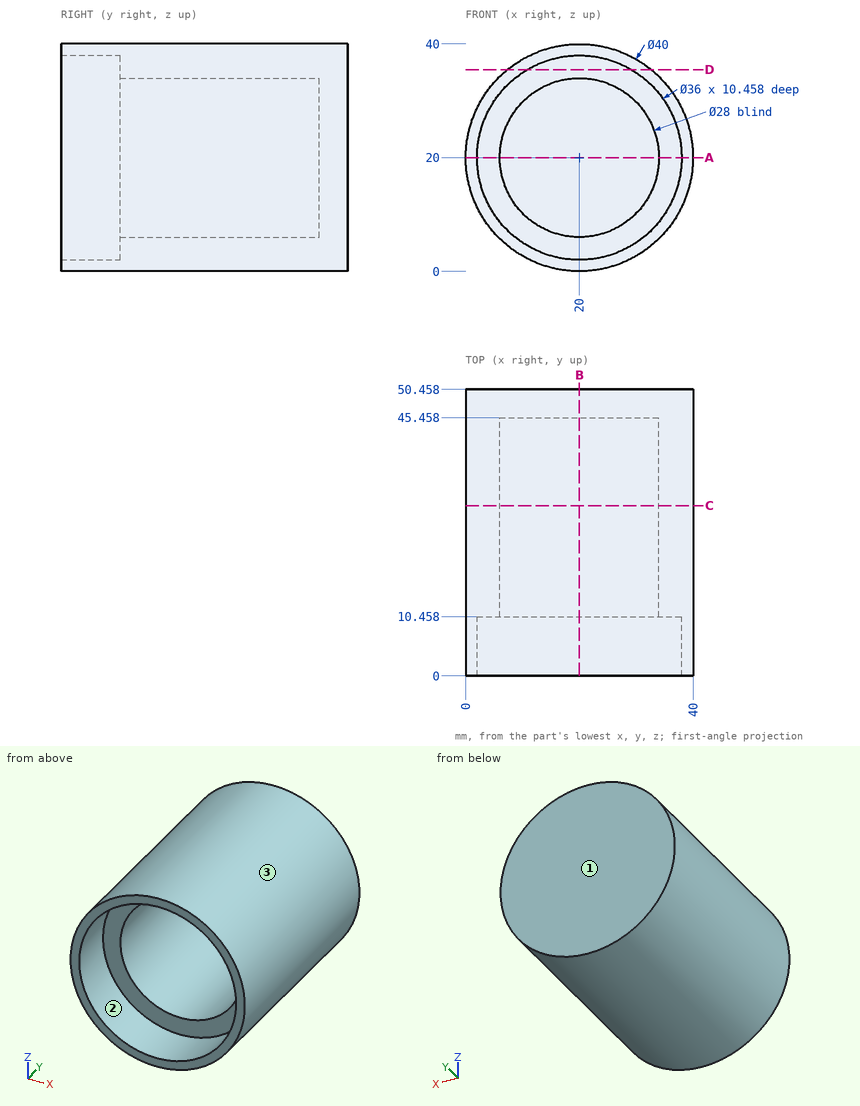
For this review, use the dimensioned drawing (mm, ordinates from the lowest corner) and the shaded views. Give positions to 0.01 mm unless a question says otherwise; leave off trailing zeros. Write each loop counter-clockwise with the first axis right and the second up, starting at its lowest first coordinate (ties: lowest second). Pieces come first, ordered by that corner, then holes. Notation, with made-up numbers: M -2.5,48 L 20.5,48 A15 ccw 20.5,69 Z; hole C -32.75,-38 d10. An arc over 180 degrees is marked long. Write item = value, one per line. Start each with the question number.
Q1. We need section D-D (z = 35.5). State the section outline as (x, y) points, plus the area to 3 significant figures.
Q2. For line 1 (X direction, y = 42, z = 20); line 2 (Y direction, x = 24.5, z = 15); line 3 (X direction, y = 13, z = 25.5), list the stretches that pass through material, from the lowest coordinate up.
Q3. Clearance check with flat-ended pins moving along their axes: pin 1 (6 mm diameter, centred on y = 42.5, z = 24, fed in from +X) (3 decimals); pin 2 (22.5 mm diameter, centred on x = 17, z = 16, fed in from -Y); pin 3 (1 mm diameter, centred on x = 11.5, z = 21, fed in from -Y). State where each tip first meets the part, or that it passes through.
Q4. We need section B-B (x = 20). State the section outline as (y, z) points, plus the area to 3 significant figures.
Q5. Mouldability with a two-part tool opening along X and no side actions: class the marked faces 1, 2 and 3 as released by +X, released by -X, zero draft, split by the parting line, or undercut.
Q6. We need section C-C (y = 30). State the section outline as (x, z) points, plus the area to 3 significant figures.
Q7. We need section A-A (z = 20). State the section outline as (x, y) points, plus the area to 3 significant figures.
Result set:
q1.outline = M 7.36,0 L 10.85,0 L 10.85,10.46 L 29.15,10.46 L 29.15,0 L 32.64,0 L 32.64,50.46 L 7.36,50.46 Z
q1.area = 1,080 mm2
q2.line_1 = 0 to 6, 34 to 40
q2.line_2 = 45.46 to 50.46
q2.line_3 = 0.77 to 7.13, 32.87 to 39.23
q3.pin_1 = 39.975
q3.pin_2 = 10.46
q3.pin_3 = 45.46
q4.outline = M 0,0 L 50.46,0 L 50.46,40 L 0,40 L 0,38 L 10.46,38 L 10.46,34 L 45.46,34 L 45.46,6 L 10.46,6 L 10.46,2 L 0,2 Z
q4.area = 662 mm2
q5.face_1 = zero draft
q5.face_2 = undercut
q5.face_3 = split by the parting line
q6.outline = C 20,20 d40; hole C 20,20 d28
q6.area = 641 mm2
q7.outline = M 0,0 L 2,0 L 2,10.46 L 6,10.46 L 6,45.46 L 34,45.46 L 34,10.46 L 38,10.46 L 38,0 L 40,0 L 40,50.46 L 0,50.46 Z
q7.area = 662 mm2
